```python
from build123d import *

# Parameters (mm, degrees)
BOSS_EXTRUDE1_DEPTH = 5
BOSS_EXTRUDE2_DEPTH = 170


with BuildPart() as part:
    # Sketch1 → Boss-Extrude1 (new body)
    with BuildSketch(Plane(origin=(0, 0, 0), x_dir=(1, 0, 0), z_dir=(0, 1, 0))):
        with BuildLine():
            Line((0, 40), (0, 12.5))
            ThreePointArc((0, 12.5), (-12.5, 0), (0, -12.5))
            Line((0, -12.5), (0, -40))
            ThreePointArc((0, -40), (-40, 0), (0, 40))
        make_face()
    extrude(amount=BOSS_EXTRUDE1_DEPTH)

    # Sketch2 → Boss-Extrude2 (add)
    with BuildSketch(Plane(origin=(0, 5, 0), x_dir=(1, 0, 0), z_dir=(0, 1, 0))):
        with BuildLine():
            ThreePointArc((-29.461839725, -24), (-38, 0), (-29.461839725, 24))
            Line((-29.461839725, 24), (-32, 24))
            ThreePointArc((-32, 24), (-40, 0), (-32, -24))
            Line((-32, -24), (-29.461839725, -24))
        make_face()
    extrude(amount=BOSS_EXTRUDE2_DEPTH)


solid = part.part
```
Could you check a few things on this model? Use its own coordinates, in mm. Round coordinates to 2 decimals unless told otherwise and drop trailing zeros. Order: outer loops, then holes, each group sorted by start corner. A loop starts at its lowest first (then second) coordinate and runs counter-clockwise, first axis right, second up. Notation, with made-up numbers: M 14.25,82.5 L 39.25,82.5 A23 cw 39.25,98.5 Z; hole C 26,8 d9. An arc over 180 degrees is marked long. One line per question, with ' | ' between items. Start each with the question number.
(1) Please list where these lines run through material, in increasing order: line 1 along Y through (x, z) = (-16.5, -22); line 2 along Z through (x, y) = (-34, 84); line 3 along Z through (x, y) = (-31, 31.5).
(2) Suppose I cut it at A-A on x = -8.5. List the corners of the cut face in (y, z) for me, then the cut area to 3 significant figures.
(3) Suppose I cut it at B-B on z = 0. List the corners of the cut face in (x, y) for me, then the cut area to 4 significant figures.
(4) Thinking about a two-plate mould opening in Z: for faces 1 (the face through (0, 2, 26)), 2 (the face through (-12.497, 2.465, -0.275)), 3 (the face through (-38, 89, 0)), 4 (the face through (-40, 81, 0)), which applies, +Z half, -Z half, draft (parallel to the pull), parting line (faces both ways), or undercut?
(5) For P1, Ø10, axis at x = -29.5, y = 20.5, coming from the +Z side; P2, Ø2, axis at x = -31.5, z = -1, coming from the +Y side; P3, Ø0.8, axis at x = -31, y = 62.5, coming from the -Z side, each with a flat end and sliding along its axis, tell me the tip position at first contact or that it passes through.
(6) Suppose I cut it at C-C on x = -24. List the corners of the cut face in (y, z) for me, then the cut area to 3 significant figures.
(7) Suppose I cut it at D-D on y = 151. List the corners of the cut face in (x, z) for me.
Geometry results:
1) line 1: 0 to 5 | line 2: -21.07 to -16.97, 16.97 to 21.07 | line 3: -24 to -21.98, 21.98 to 24
2) outline: M 0,-39.09 L 5,-39.09 L 5,-9.17 L 0,-9.17 Z; M 0,9.17 L 5,9.17 L 5,39.09 L 0,39.09 Z | area: 299 mm²
3) outline: M -40,0 L -12.5,0 L -12.5,5 L -38,5 L -38,175 L -40,175 Z | area: 477.5 mm²
4) face 1: draft | face 2: undercut | face 3: undercut | face 4: parting line
5) P1: z = 24 | P2: y = 5 | P3: z = -24
6) outline: M 0,-32 L 5,-32 L 5,32 L 0,32 Z | area: 320 mm²
7) outline: M -32,-24 L -29.46,-24 A38 cw -29.46,24 L -32,24 A40 ccw Z
